For this review, use the dimensioned drawing (mm, ordinates from the lowest corner) and the shaded views. A direction names the side the tool comes from. Round coordinates to 2 decimals unless told otherwise and drop trailing zeros. Write each loop counter-clockwise with the first axis right and the second up, starting at its lowest first coordinate (ties: lowest second). Pieces come first, ordered by that corner, then holes. Notation, with made-up numbers: M -13.5,-21 L 33.5,-21 A6 cw 33.5,-17 Z; hole C 79,7 d8. An arc over 180 degrees is marked long. Use one line per item in the form item = value. Start each with the question number.
Item 1: Add section A-A (x = 17). State the section outline as (y, z) points.
Item 2: For line 1 (Y direction, x = 16.5, z = 7.25); line 2 (X direction, y = 3, z = 5); line 3 (Z direction, x = 21.25, y = 30), list the stretches that pass through material, from the lowest coordinate up. Write a range as [from, to].
Item 3: For the marked faces 4 and 5, list the 3-axis set-ups (+Z, -Z, +X, -X, +Y, -Y) from which the entire face can be reached by the end or side of a thin tool; tool diameter is ignored.
Item 4: Add section B-B (z = 6.75). State the section outline as (x, y) points.
Item 5: Draft analysis for pull direction Y (two halves, no side actions). For the marked faces 1, 2 and 3, state which applies: released by +Y, released by -Y, zero draft, split by the parting line, or undercut.
Item 6: Add section C-C (y = 2). State the section outline as (x, z) points.
Item 7: Add section D-D (x = 21). State the section outline as (y, z) points, and give its area (3 significant figures).
Item 8: For P1, Ø1, axis at y = 17, z = 10.5, coming from the -X side; P2, Ø1.5, axis at y = 34.5, z = 6, coming from the +X side; P3, Ø1.5, axis at x = 23.5, y = 24.5, coming from the -Z side, all flat-tipped, find the tip position at first contact; note any pin that passes through.
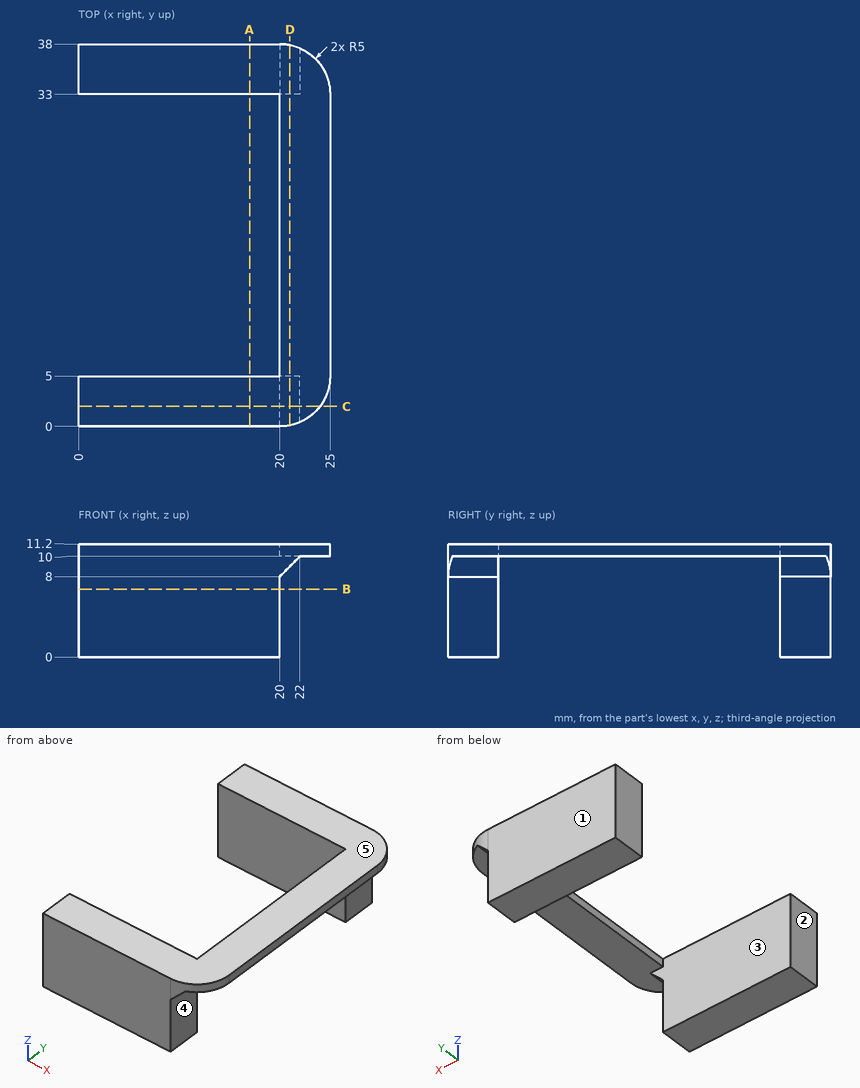
Calculated:
q1.outline = M 0,0 L 5,0 L 5,11.2 L 0,11.2 Z; M 33,0 L 38,0 L 38,11.2 L 33,11.2 Z
q2.line_1 = [0, 5], [33, 38]
q2.line_2 = [0, 20]
q2.line_3 = [10, 11.2]
q3.face_4 = -Z, +X, +Y, -Y
q3.face_5 = +Z, +X, -X, +Y, -Y
q4.outline = M 0,0 L 20,0 L 20,5 L 0,5 Z; M 0,33 L 20,33 L 20,38 L 0,38 Z
q5.face_1 = released by +Y
q5.face_2 = zero draft
q5.face_3 = undercut
q6.outline = M 0,0 L 20,0 L 20,8 L 22,10 L 24,10 L 24,11.2 L 0,11.2 Z
q7.outline = M 0.1,9 L 5,9 L 5,10 L 33,10 L 33,9 L 37.9,9 L 37.9,11.2 L 0.1,11.2 Z
q7.area = 55.2 mm^2
q8.P1 = 20
q8.P2 = 20
q8.P3 = 10
